Source: CAD feature listing. Evaluate the final solid. Frame: model axes, mm. Face numbers are marked on the shaded views. A direction names the side the tool comes from. Coordinates: 2 decimals unless noted, no trailing zeros. Order: outer loops, then holes, each group sorted by start corner. A loop starts at its lowest first (then second) coordinate and runs counter-clockwise, first axis right, second up. Notation, with made-up numbers: (2.5, 21.25) -> (31.5, 21.25) arc R25 cw to (31.5, 53.25) -> close; hole circle Ø11 at (48, 67). An arc over 180 degrees is marked (long way). Write item = value, one per line. Start each with the question number.
Item 1: Section query A-A (y = 0). Count the separate pieces of the cut face and the enclosed holes in it, then the cut area to 3 significant figures.
Item 2: Contact query for flat-ended pins moving along their axis: pin 1 (10 mm diameter, centred on y = -6, z = -13.5, fed in from +X); pin 2 (2 mm diameter, centred on x = 50, z = -9, fed in from +Y); pin 3 (9 mm diameter, centred on y = 2, z = -16.5, fed in from -X); pin 4 (1.2 mm diameter, centred on x = 2.5, y = 0, fed in from +Z). Output: stop coordinate, or through.
Item 3: Set-up query: the marked faces 1, 2, 3, 4 and 5. Return all of +Z, -Z, +X, -X, +Y, -Y with unobstructed straight access to the full face (end or side cutting, diameter ignored); none if empty.
Item 4: Mould query, pull axis X, two halves, no side actions, for the marked faces 6 and 7. Classes: released by +X, released by -X, zero draft, split by the parting line, or undercut.
Item 5: Section query C-C (x = 2.5). Output: boundary loops of the cut face in (y, z).
Item 6: Section query D-D (x = 49). Output: boundary loops of the cut face in (y, z) (3 decimals).
Item 7: Ray query, line 1 along Z through (x, y) = (21.5, -16.5); line 2 along Z through (x, y) = (43, 0); line 3 along Y through (x, z) = (79, -6.5). Return the intervals inside material, ascending. Write a range as [from, to].
```python
from build123d import *

# Parameters (mm, degrees)
BOSS_EXTRU_1_DEPTH           = 114
ESQUISSE2_R                  = 22.55
ENL_V_MAT_EXTRU_2_DEPTH      = 5
ENL_V_START                  = -5
ESQUISSE4_R                  = 22.55
ENL_V_MAT_EXTRU_3_DEPTH      = 5
ESQUISSE5_R                  = 1
ENL_V_MAT_EXTRU_4_DEPTH      = 118.883477756
BOSS_EXTRU_2_START           = -2
BOSS_EXTRU_2_DEPTH           = 2
BOSS_EXTRU_3_START           = 9
BOSS_EXTRU_3_DEPTH           = 9
BOSS_EXTRU_4_START           = 2
BOSS_EXTRU_4_DEPTH           = 2
BOSS_EXTRU_5_START           = -2
BOSS_EXTRU_5_DEPTH           = 2
BOSS_EXTRU_6_START           = 9
BOSS_EXTRU_6_DEPTH           = 9
BOSS_EXTRU_7_START           = 2
BOSS_EXTRU_7_DEPTH           = 2
ESQUISSE12_W                 = 13.751826503
ESQUISSE12_H                 = 1
ESQUISSE12_W_2               = 11.167500513
ENL_V_MAT_EXTRU_5_DEPTH      = 95.05366831
BOSS_EXTRU_8_START           = -13
BOSS_EXTRU_8_DEPTH           = 13
BOSS_EXTRU_9_START           = -13
BOSS_EXTRU_9_DEPTH           = 13
ENL_V_MAT_EXTRU_6_DEPTH      = 94.846110875
ENL_V_MAT_EXTRU_7_DEPTH      = 119.048305907
ENL_V_MAT_EXTRU_7_DEPTH_BACK = 119.048305907
ESQUISSE16_R                 = 2


with BuildPart() as part:
    # Esquisse1 → Boss.-Extru.1 (new body)
    with BuildSketch(Plane(origin=(0, 0, 0), x_dir=(0, 0, -1), z_dir=(1, 0, 0))):
        with BuildLine():
            Line((14.144270925, 14.14), (17.975320492, 17.947474134))
            ThreePointArc((17.975320492, 17.947474134), (24.05, 0), (17.975320492, -17.947474134))
            Line((17.975320492, -17.947474134), (14.144270925, -14.14))
            ThreePointArc((14.144270925, -14.14), (20, 0), (14.144270925, 14.14))
        make_face()
    extrude(amount=BOSS_EXTRU_1_DEPTH)

    # Esquisse2 → Enlèv. mat.-Extru.2 (cut)
    with BuildSketch(Plane.ZY):
        Circle(ESQUISSE2_R)
    extrude(amount=-ENL_V_MAT_EXTRU_2_DEPTH, mode=Mode.SUBTRACT)

    # Esquisse4 → Enlèv. mat.-Extru.3 (cut)
    with BuildSketch(Plane(origin=(114, 0, 0), x_dir=(0, 0, -1), z_dir=(1, 0, 0)).offset(ENL_V_START)):
        Circle(ESQUISSE4_R)
    extrude(amount=ENL_V_MAT_EXTRU_3_DEPTH, mode=Mode.SUBTRACT)

    # Esquisse5 → Enlèv. mat.-Extru.4 (cut, through all)
    with BuildSketch(Plane.XY):
        with Locations((2.5, 0)):
            Circle(ESQUISSE5_R)
        with Locations((111.5, 0)):
            Circle(ESQUISSE5_R)
    extrude(amount=-ENL_V_MAT_EXTRU_4_DEPTH, mode=Mode.SUBTRACT)

    # Esquisse6 → Boss.-Extru.2 (add)
    with BuildSketch(Plane(origin=(88.7, 0, 0), x_dir=(0, 0, -1), z_dir=(1, 0, 0)).offset(BOSS_EXTRU_2_START)):
        with BuildLine():
            Line((0, 17), (0, 20))
            ThreePointArc((0, 20), (20, 0), (0, -20))
            Line((0, -20), (0, -17))
            ThreePointArc((0, -17), (17, 0), (0, 17))
        make_face()
    extrude(amount=BOSS_EXTRU_2_DEPTH)

    # Esquisse7 → Boss.-Extru.3 (add)
    with BuildSketch(Plane.ZY.offset(-86.7).offset(BOSS_EXTRU_3_START)):
        with BuildLine():
            Line((0, 20), (0, 19))
            ThreePointArc((0, 19), (-19, 0), (0, -19))
            Line((0, -19), (0, -20))
            ThreePointArc((0, -20), (-20, 0), (0, 20))
        make_face()
    extrude(amount=-BOSS_EXTRU_3_DEPTH)

    # Esquisse8 → Boss.-Extru.4 (add)
    with BuildSketch(Plane.ZY.offset(-77.7).offset(BOSS_EXTRU_4_START)):
        with BuildLine():
            Line((0, 20), (0, 18))
            ThreePointArc((0, 18), (-18, 0), (0, -18))
            Line((0, -18), (0, -20))
            ThreePointArc((0, -20), (-20, 0), (0, 20))
        make_face()
    extrude(amount=-BOSS_EXTRU_4_DEPTH)

    # Esquisse9 → Boss.-Extru.5 (add)
    with BuildSketch(Plane(origin=(55.6, 0, 0), x_dir=(0, 0, -1), z_dir=(1, 0, 0)).offset(BOSS_EXTRU_5_START)):
        with BuildLine():
            Line((0, 20), (0, 17))
            ThreePointArc((0, 17), (17, 0), (0, -17))
            Line((0, -17), (0, -20))
            ThreePointArc((0, -20), (20, 0), (0, 20))
        make_face()
    extrude(amount=BOSS_EXTRU_5_DEPTH)

    # Esquisse10 → Boss.-Extru.6 (add)
    with BuildSketch(Plane.ZY.offset(-53.6).offset(BOSS_EXTRU_6_START)):
        with BuildLine():
            Line((0, 20), (0, 19))
            ThreePointArc((0, 19), (-19, 0), (0, -19))
            Line((0, -19), (0, -20))
            ThreePointArc((0, -20), (-20, 0), (0, 20))
        make_face()
    extrude(amount=-BOSS_EXTRU_6_DEPTH)

    # Esquisse11 → Boss.-Extru.7 (add)
    with BuildSketch(Plane.ZY.offset(-44.6).offset(BOSS_EXTRU_7_START)):
        with BuildLine():
            Line((0, 20), (0, 18))
            ThreePointArc((0, 18), (-18, 0), (0, -18))
            Line((0, -18), (0, -20))
            ThreePointArc((0, -20), (-20, 0), (0, 20))
        make_face()
    extrude(amount=-BOSS_EXTRU_7_DEPTH)

    # Esquisse12 → Enlèv. mat.-Extru.5 (cut, through all)
    with BuildSketch(Plane(origin=(88.7, 0, 0), x_dir=(0, 0, -1), z_dir=(1, 0, 0))):
        with Locations((6.875913252, -19.5)):
            Rectangle(ESQUISSE12_W, ESQUISSE12_H)
        with Locations((5.583750257, 19.5)):
            Rectangle(ESQUISSE12_W_2, ESQUISSE12_H)
    extrude(amount=-ENL_V_MAT_EXTRU_5_DEPTH, mode=Mode.SUBTRACT)

    # Esquisse13 → Boss.-Extru.8 (add)
    with BuildSketch(Plane(origin=(88.7, 0, 0), x_dir=(0, 0, -1), z_dir=(1, 0, 0)).offset(BOSS_EXTRU_8_START)):
        with BuildLine():
            Line((17.975320492, 17.947474134), (14.144270925, 14.14))
            ThreePointArc((14.144270925, 14.14), (10.480241973, 17.034216395), (6.244997998, 19))
            Line((6.244997998, 19), (17.4396757, 18.627232183))
            ThreePointArc((17.4396757, 18.627232183), (17.709986765, 18.289314213), (17.975320492, 17.947474134))
        make_face()
        with BuildLine():
            Line((14.144270925, -14.14), (17.975320492, -17.947474134))
            ThreePointArc((17.975320492, -17.947474134), (17.559611782, -18.478549847), (17.131891216, -19))
            Line((17.131891216, -19), (6.244997998, -19))
            ThreePointArc((6.244997998, -19), (10.480241973, -17.034216395), (14.144270925, -14.14))
        make_face()
    extrude(amount=BOSS_EXTRU_8_DEPTH)

    # Esquisse14 → Boss.-Extru.9 (add)
    with BuildSketch(Plane(origin=(55.6, 0, 0), x_dir=(0, 0, -1), z_dir=(1, 0, 0)).offset(BOSS_EXTRU_9_START)):
        with BuildLine():
            Line((14.144270925, 14.14), (17.975320492, 17.947474134))
            ThreePointArc((17.975320492, 17.947474134), (17.709986765, 18.289314213), (17.4396757, 18.627232183))
            Line((17.4396757, 18.627232183), (6.244997998, 19))
            ThreePointArc((6.244997998, 19), (10.480241973, 17.034216395), (14.144270925, 14.14))
        make_face()
        with BuildLine():
            Line((14.144270925, -14.14), (17.975320492, -17.947474134))
            ThreePointArc((17.975320492, -17.947474134), (17.559611782, -18.478549847), (17.131891216, -19))
            Line((17.131891216, -19), (6.244997998, -19))
            ThreePointArc((6.244997998, -19), (10.480241973, -17.034216395), (14.144270925, -14.14))
        make_face()
    extrude(amount=BOSS_EXTRU_9_DEPTH)

    # Esquisse15 → Enlèv. mat.-Extru.6 (cut, through all)
    with BuildSketch(Plane(origin=(88.7, 0, 0), x_dir=(0, 0, -1), z_dir=(1, 0, 0))):
        with BuildLine():
            Line((14.409304815, 20.298729325), (16.901493379, 24.760797344))
            Line((16.901493379, 24.760797344), (24.890475951, 20.298729325))
            Line((24.890475951, 20.298729325), (20.895984665, 15.394026057))
            ThreePointArc((20.895984665, 15.394026057), (17.822174246, 18.070587713), (14.409304815, 20.298729325))
        make_face()
        with BuildLine():
            Line((14.409304815, -20.298729325), (16.901493379, -24.760797344))
            Line((16.901493379, -24.760797344), (22.934233847, -18.464332541))
            Line((22.934233847, -18.464332541), (20.431131458, -15.848802481))
            ThreePointArc((20.431131458, -15.848802481), (17.561732891, -18.265269573), (14.409304815, -20.298729325))
        make_face()
    extrude(amount=-ENL_V_MAT_EXTRU_6_DEPTH, mode=Mode.SUBTRACT)

    # Esquisse16 → Enlèv. mat.-Extru.7 (cut, two sides: drawn at the far end of the back side and taken through both)
    with BuildSketch(Plane.XY.offset(-ENL_V_MAT_EXTRU_7_DEPTH_BACK)):
        with Locations((114, 13)):
            Circle(ESQUISSE16_R)
        with Locations((114, -13)):
            Circle(ESQUISSE16_R)
    extrude(amount=ENL_V_MAT_EXTRU_7_DEPTH + ENL_V_MAT_EXTRU_7_DEPTH_BACK, mode=Mode.SUBTRACT)


solid = part.part
```
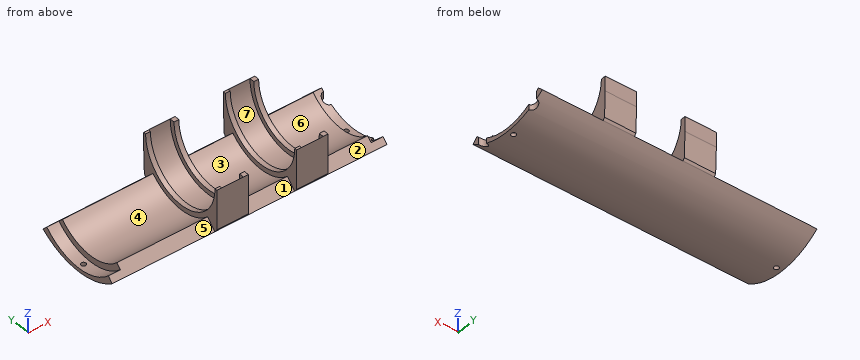
Computed:
q1.separate_pieces = 3
q1.enclosed_holes = 0
q1.area = 468 mm^2
q2.pin_1 = 88.7
q2.pin_2 = 18.94
q2.pin_3 = 5
q2.pin_4 = through
q3.face_1 = +Z, -Y
q3.face_2 = +Z, +X, -Y
q3.face_3 = +Z
q3.face_4 = +Z, -X
q3.face_5 = +Z, -X, -Y
q4.face_6 = zero draft
q4.face_7 = undercut
q5.outline = (-17.95, -17.98) arc R29.55 ccw to (-1, -24.03) -> (-1, -22.53) arc R22.55 cw to (-15.94, -15.95) -> close; (1, -24.03) arc R29.55 ccw to (17.95, -17.98) -> (15.94, -15.95) arc R22.55 cw to (1, -22.53) -> close
q6.outline = (-19, -16.521) arc R29.55 ccw to (-17.963, -17.963) arc R29.55 ccw to (-17.947, -17.975) arc R29.55 ccw to (17.947, -17.975) arc R29.55 ccw to (17.963, -17.963) arc R29.55 ccw to (18.64, -17.042) -> (19, -6.245) -> (19, 0) arc R19 cw to (-19, 0) -> close
q7.line_1 = [-19.01, -16.52]
q7.line_2 = [-24.05, -18]
q7.line_3 = [-19, -17.85], [17.85, 18.99]
